```python
from build123d import *

# Parameters (mm, degrees)
SKETCH1_R           = 6.35
BOSS_EXTRUDE1_DEPTH = 24.7
SKETCH3_R           = 1.13
CUT_EXTRUDE1_DEPTH  = 28.253825364


with BuildPart() as part:
    # Sketch1 → Boss-Extrude1 (new body)
    with BuildSketch(Plane(origin=(0, 0, 0), x_dir=(1, 0, 0), z_dir=(0, 1, 0))):
        with Locations(Location((0, 0, 0), (0, 0, 270))):
            Circle(SKETCH1_R)
        with BuildLine():
            Line((-2.742383206, -3.260332823), (2.742383206, -3.260332823))
            ThreePointArc((2.742383206, -3.260332823), (0, 4.260332823), (-2.742383206, -3.260332823))
        make_face(mode=Mode.SUBTRACT)
    extrude(amount=BOSS_EXTRUDE1_DEPTH)

    # Sketch3 → Cut-Extrude1 (cut, through all)
    with BuildSketch(Plane(origin=(0, 0, 3.260332823), x_dir=(-1, 0, 0), z_dir=(0, 0, -1))):
        with Locations((0, 18.35)):
            Circle(SKETCH3_R)
        with Locations(Location((0, 6.35, 0), (0, 0, 270))):
            Circle(SKETCH3_R)
    extrude(amount=-CUT_EXTRUDE1_DEPTH, mode=Mode.SUBTRACT)


solid = part.part
```
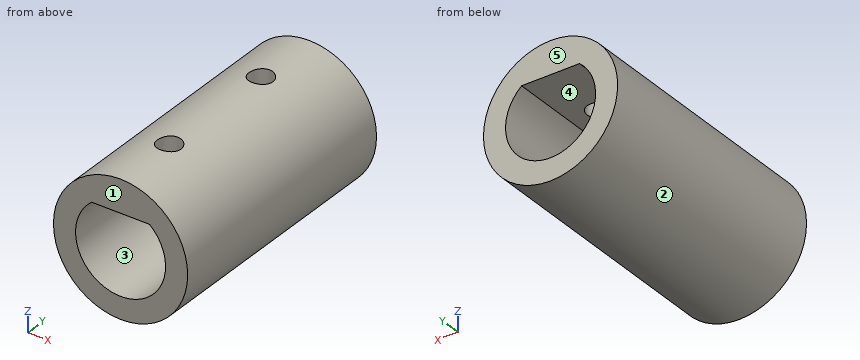
Model file for the job. Use its own axes, mm. Face numbers are marked on the shaded views. A direction names the side the tool comes from. Give positions to 0.01 mm unless a question says otherwise; leave off trailing zeros. Write each loop counter-clockwise with the first axis right and the second up, starting at its lowest first coordinate (ties: lowest second). Pieces come first, ordered by that corner, then holes. Notation, with made-up numbers: (76.5, -11.75) -> (127.5, -11.75) arc R32 cw to (127.5, 22.25) -> close; hole circle Ø2 at (15.5, -11.5). An arc over 180 degrees is marked (long way). Use CSV: the item, a comma, the result in double quotes. Start each with the question number.
1) Two-plate mould, pull along X, no slides. Class the marked faces 1, 2 and 3: released by +X, released by -X, zero draft, split by the parting line, or undercut.
2) Cut at B-B on z = 0. List the corners of the cut face in (x, y).
3) Cut at A-A on x = 0. List the corners of the cut face in (y, z).
4) Cut at C-C on x = -1.75. List the corners of the cut face in (y, z), plus the area to 3 significant figures.
5) Drill centre lines: L1, parallel to Y at x = 0, z = 5.35; L2, parallel to Y at x = -1, z = 4.5; L3, parallel to X at y = 6.35, z = 4.8. Where is each one in solid material? Low to high.
6) Tool access for the marked faces 4 and 5: list every direction of +Z, -Z, +X, -X, +Y, -Y with a clear straight run to the whole face (end or side of a thin tool).
7) Pin check, flat tips, straight feed: P1, Ø4, axis at x = 4, y = 15, coming from the +Z side; P2, Ø1, axis at x = 1, z = -2, coming from the -Y side; P3, Ø2, axis at x = 0, y = 6.35, coming from the +Z side. Stop position of each tip, or through.
8) Cut at D-D on y = 22.75. List the corners of the cut face in (x, z).
Final values:
1,face 1,"zero draft"
1,face 2,"split by the parting line"
1,face 3,"undercut"
2,outline,"(-6.35, 0) -> (-4.26, 0) -> (-4.26, 24.7) -> (-6.35, 24.7) -> close; (4.26, 0) -> (6.35, 0) -> (6.35, 24.7) -> (4.26, 24.7) -> close"
3,outline,"(0, -6.35) -> (24.7, -6.35) -> (24.7, -4.26) -> (0, -4.26) -> close; (0, 3.26) -> (5.22, 3.26) -> (5.22, 6.35) -> (0, 6.35) -> close; (7.48, 3.26) -> (17.22, 3.26) -> (17.22, 6.35) -> (7.48, 6.35) -> close; (19.48, 3.26) -> (24.7, 3.26) -> (24.7, 6.35) -> (19.48, 6.35) -> close"
4,outline,"(0, -6.1) -> (24.7, -6.1) -> (24.7, -3.88) -> (0, -3.88) -> close; (0, 3.26) -> (24.7, 3.26) -> (24.7, 6.1) -> (0, 6.1) -> close"
4,area,"125 mm2"
5,L1,"y = 0 to 5.22, 7.48 to 17.22, 19.48 to 24.7"
5,L2,"y = 0 to 5.82, 6.88 to 17.82, 18.88 to 24.7"
5,L3,"x = -4.16 to -1.13, 1.13 to 4.16"
6,face 4,"+Y, -Y"
6,face 5,"+Z, -Z, +X, -X, +Y"
7,P1,"stops at z = 6.03"
7,P2,"passes through"
7,P3,"stops at z = -4.14"
8,outline,"circle Ø12.7 at (0, 0); hole (-2.74, 3.26) arc R4.26 ccw (long way) to (2.74, 3.26) -> close"
